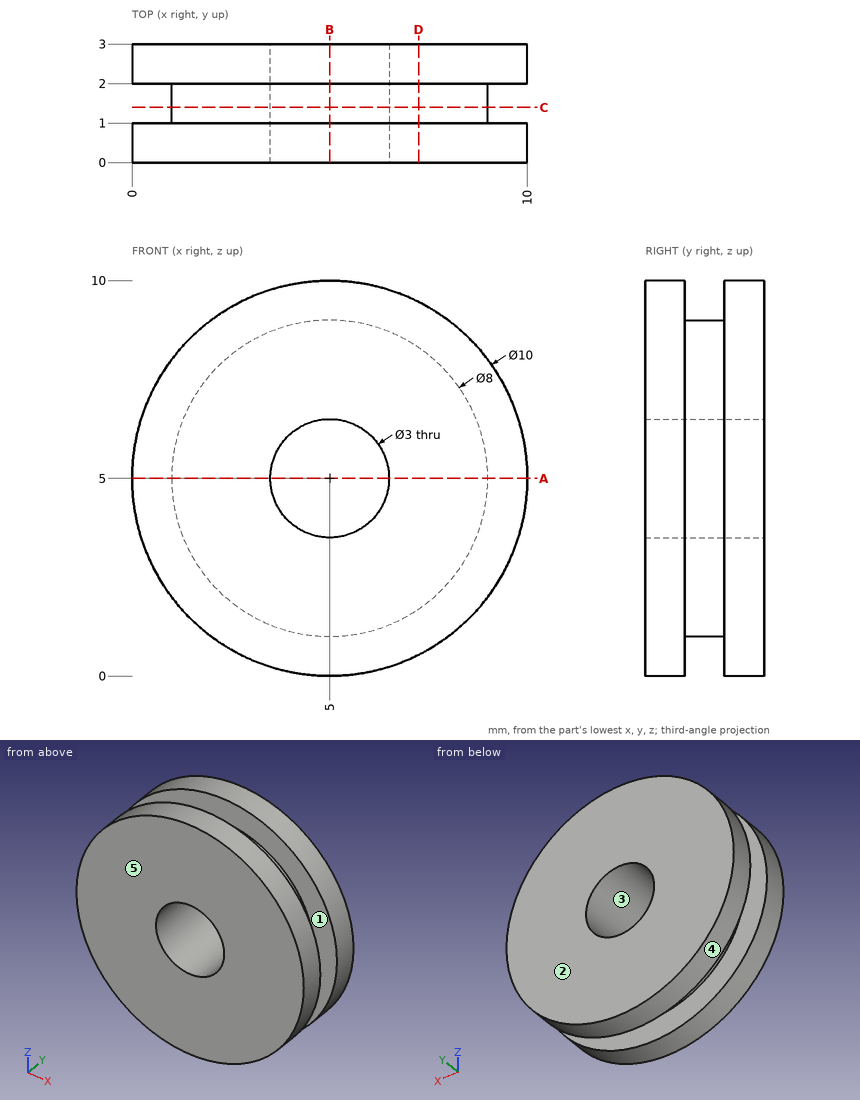
Job drawing, mm, ordinate dimensions from the low corner. One solid piece. A direction names the side the tool comes from. Round coordinates to 2 decimals unless told otherwise and drop trailing zeros. Loops run counter-clockwise (first coordinate to the right, second up) from the corner with the lowest first, then second, coordinate; pieces in that order, holes last. Notation, with made-up numbers: (41.25, -28) -> (95.25, -28) arc R34 ccw to (95.25, 11) -> close; hole circle Ø1 at (46, 49). An arc over 180 degrees is marked (long way). Use a Markdown table: item, result.
1) Cut at D-D, the plane x = 7.25. List the corners of the cut face in (y, z), and give its area (3 significant figures).
The answers:
| item | result |
|---|---|
| outline | (0, 0.53) -> (1, 0.53) -> (1, 1.69) -> (2, 1.69) -> (2, 0.53) -> (3, 0.53) -> (3, 9.47) -> (2, 9.47) -> (2, 8.31) -> (1, 8.31) -> (1, 9.47) -> (0, 9.47) -> close |
| area | 24.5 mm2 |
2) Cut at B-B, the plane x = 5. List the corners of the cut face in (y, z).
The answers:
| item | result |
|---|---|
| outline | (0, 0) -> (1, 0) -> (1, 1) -> (2, 1) -> (2, 0) -> (3, 0) -> (3, 3.5) -> (0, 3.5) -> close; (0, 6.5) -> (3, 6.5) -> (3, 10) -> (2, 10) -> (2, 9) -> (1, 9) -> (1, 10) -> (0, 10) -> close |
3) Tool access for the marked faces 1 and 2: list every direction of +Z, -Z, +X, -X, +Y, -Y with a clear straight run to the whole face (end or side of a thin tool).
The answers:
| item | result |
|---|---|
| face 1 | none |
| face 2 | +Z, -Z, +X, -X, +Y |
4) Drop flat-ended pins along their axis: pin 1 Ø6 at (x, z) = (7.5, 3.5) entering from -Y; pin 2 Ø1.8 at (x, z) = (5, 5) entering from +Y. Give the stop position or say it passes through.
The answers:
| item | result |
|---|---|
| pin 1 | stops at y = 0 |
| pin 2 | passes through |
5) Probe line 1 (Y direction, x = 4.5, z = 9); line 2 (X direction, y = 1.8, z = 5). List the from-to ranges inside material, lowest first. Write a range as [from, to].
The answers:
| item | result |
|---|---|
| line 1 | y = [0, 1], [2, 3] |
| line 2 | x = [1, 3.5], [6.5, 9] |
6) Pull direction Z, two halves, no side cores. Call the marked faces 3, 4 and 5: pulls with the +Z half, pulls with the -Z half, needs draft (parallel to the pull), parting line crosses it, or undercut.
The answers:
| item | result |
|---|---|
| face 3 | undercut |
| face 4 | parting line crosses it |
| face 5 | needs draft |
7) Cut at A-A, the plane z = 5. List the corners of the cut face in (x, y), and give its area (3 significant figures).
The answers:
| item | result |
|---|---|
| outline | (0, 0) -> (3.5, 0) -> (3.5, 3) -> (0, 3) -> (0, 2) -> (1, 2) -> (1, 1) -> (0, 1) -> close; (6.5, 0) -> (10, 0) -> (10, 1) -> (9, 1) -> (9, 2) -> (10, 2) -> (10, 3) -> (6.5, 3) -> close |
| area | 19.0 mm2 |
8) Cut at C-C, the plane y = 1.4. List the corners of the cut face in (x, z).
The answers:
| item | result |
|---|---|
| outline | circle Ø8 at (5, 5); hole circle Ø3 at (5, 5) |
